Autodesk Inventor part; units mm, degrees
ref_plane "YZ Plane" through (0, 0, 0) normal (1, 0, 0) x (0, 1, 0)
ref_plane "XZ Plane" through (0, 0, 0) normal (0, 1, 0) x (-1, 0, 0)
ref_plane "XY Plane" through (0, 0, 0) normal (0, 0, 1) x (1, 0, 0)
sketch "Sketch1" plane through (0, 0, 0) normal (0, 1, 0) x (-1, 0, 0)
  circle A0 centre (-9, 0) radius 8.5
  circle A1 centre (15, 0) radius 4
  line L0 (10.6066, -10.6066) -> (17.9306, -2.7224)
  line L1 (10.6066, 10.6066) -> (17.9306, 2.7224)
  line L2 (16.6, -2.7713) -> (13.4, -2.7713)
  line L3 (13.4, -2.7713) -> (11.8, 0)
  line L4 (11.8, 0) -> (13.4, 2.7713)
  line L5 (13.4, 2.7713) -> (16.6, 2.7713)
  line L6 (16.6, 2.7713) -> (18.2, 0)
  line L7 (18.2, 0) -> (16.6, -2.7713)
  line L8 (15, -2.7713) -> (15, 2.7713)
  line L9 (11.8, 0) -> (15, 0)
  circle A2 centre (-9, 0) radius 6
  circle A3 centre (-9, -6) radius 1.2
  circle A4 centre (-15, 0) radius 1.2
  circle A5 centre (-9, 6) radius 1.2
  circle A6 centre (-3, 0) radius 1.2
  circle A7 centre (15, 0) radius 1.65
  line L10 (11, 0) -> (-29, 0)
  circle A8 centre (-33, 0) radius 4
  line L11 (-28.6066, -10.6066) -> (-35.9306, -2.7224)
  line L12 (-28.6066, 10.6066) -> (-35.9306, 2.7224)
  line L13 (-31.4, -2.7713) -> (-34.6, -2.7713)
  line L14 (-34.6, -2.7713) -> (-36.2, 0)
  line L15 (-36.2, 0) -> (-34.6, 2.7713)
  line L16 (-36.2, 0) -> (-33, 0)
  line L17 (-33, -2.7713) -> (-33, 2.7713)
  line L18 (-34.6, 2.7713) -> (-31.4, 2.7713)
  line L19 (-29.8, 0) -> (-31.4, -2.7713)
  line L20 (-31.4, 2.7713) -> (-29.8, 0)
  circle A9 centre (-33, 0) radius 1.65
  line L21 (-28.6066, -10.6066) -> (10.6066, -10.6066)
  line L22 (-28.6066, 10.6066) -> (10.6066, 10.6066)
  dimension "d49" = 4
  dimension "d55" = 8
  dimension "d22" = 3.2
  dimension "d34" = 12
  dimension "d35" = 2.4
  dimension "d36" = 2.4
  dimension "d37" = 2.4
  dimension "d38" = 2.4
  dimension "d43" = 3.3
  dimension "d54" = 40
  dimension "d56" = 3.2
  dimension "d57" = 3.2
  dimension "d58" = 120
  dimension "d59" = 3.2
  dimension "d60" = 120
  dimension "d61" = 3.3
extrude "Extrusion1" add sketch "Sketch1" along normal blind 10 contours L10 A6 A2 A5 A4 A0 | L10 A1 L0 L21 L11 A8 A0 | A0 L10 A8 L12 L22 L1 A1 | A0 L10 A4 A2 A3 A6 | A1 | L10 A2 A6 | A6 A2 L10 | L10 A2 A4 | A4 A2 L10 | A8 | A6 L10 A4 A2 A5 | A2 L10 A6 | A6 L10 A2 | A2 A3 A4 L10 A6 | A4 L10 A2 | A2 L10 A4 | A5 A2 | A2 A5 | A3 A2 | A2 A3 | L2 L8 A7 L5 L6 L7 | L2 L3 L9 A7 L8 | A7 L9 L8 | L8 A7 | L4 L5 L8 A7 L9 | L9 A7 L8 | L13 L17 A9 L18 L20 L19 | L13 L14 L16 A9 L17 | A9 L16 L17 | L17 A9 | L15 L18 L17 A9 L16 | L16 A9 L17
extrude "Extrusion2" cut sketch "Sketch1" along normal blind 2.5 contours L10 A6 A2 A5 A4 A0 | A0 L10 A4 A2 A3 A6 | L10 A2 A6 | A6 A2 L10 | L10 A2 A4 | A4 A2 L10 | A6 L10 A4 A2 A5 | A2 L10 A6 | A6 L10 A2 | A2 A3 A4 L10 A6 | A4 L10 A2 | A2 L10 A4 | A5 A2 | A2 A5 | A3 A2 | A2 A3 | L2 L8 A7 L5 L6 L7 | L2 L3 L9 A7 L8 | A7 L9 L8 | L8 A7 | L4 L5 L8 A7 L9 | L9 A7 L8 | L13 L17 A9 L18 L20 L19 | L13 L14 L16 A9 L17 | A9 L16 L17 | L17 A9 | L15 L18 L17 A9 L16 | L16 A9 L17
extrude "Extrusion3" cut sketch "Sketch1" along normal blind 10 contours L10 A2 A6 | A6 A2 L10 | L10 A2 A4 | A4 A2 L10 | A2 L10 A6 | A6 L10 A2 | A4 L10 A2 | A2 L10 A4 | A5 A2 | A2 A5 | A3 A2 | A2 A3 | A7 L9 L8 | L8 A7 | L9 A7 L8 | A9 L16 L17 | L17 A9 | L16 A9 L17
fillet "Fillet1" radius 0.3 20 edges at (-19, 0, 0) (-14.2686, 0, 6.6645) (-14.2686, 0, -6.6645) (-19, 10, 0) (-14.2686, 10, 6.6645) (-14.2686, 10, -6.6645) (9, 10, 10.6066) (9, 0, 10.6066) (9, 10, -10.6066) (9, 0, -10.6066) (-10.6066, 5, -10.6066) (-10.6066, 5, 10.6066) (37, 0, 0) (32.2686, 0, -6.6645) (32.2686, 0, 6.6645) (37, 10, 0) (32.2686, 10, -6.6645) (32.2686, 10, 6.6645) (28.6066, 5, -10.6066) (28.6066, 5, 10.6066)
sketch "Sketch2" plane through (0, 10, 0) normal (0, 1, 0) x (1, 0, 0)
  circle A0 centre (3, 0) radius 1.2
  circle A1 centre (3, 0) radius 2
  circle A2 centre (9, 6) radius 1.2
  circle A3 centre (9, 6) radius 2
  circle A4 centre (15, 0) radius 1.2
  circle A5 centre (15, 0) radius 2
  circle A6 centre (9, -6) radius 1.2
  circle A7 centre (9, -6) radius 2
  point P0 (0, 0)
  dimension "d22" = 3.2
  dimension "d43" = 3.3
  dimension "d48" = 4
  dimension "d49" = 4
  dimension "d50" = 4
  dimension "d51" = 4
extrude "Extrusion5" cut sketch "Sketch2" against normal blind 2 contours A0 | A1 | A2 | A3 | A4 | A5 | A6 | A7
properties part number "neck_v2"
Input: part model. Units: mm. Frame: model coordinates. A direction names the side the tool comes from. Coordinates: 2 decimals unless noted, no trailing zeros. Write each loop counter-clockwise with the first axis right and the second up, starting at its lowest first coordinate (ties: lowest second). Pieces come first, ordered by that corner, then holes.
1) Section D-D on y = 8.5. Output: boundary loops of the cut face in (x, z).
2) Section B-B on y = 6.25. Output: boundary loops of the cut face in (x, z), and give its area (4 significant figures).
3) Section A-A on x = 9. Output: boundary loops of the cut face in (y, z), and give its area (3 significant figures).
4) Material intervals for line 1 along Z through (x, y) = (9, 5.5); line 2 along Z through (x, y) = (3, 6.2); line 3 along Y through (x, z) = (4, -5.75), sorted ascending.
5) Mould query, pull axis X, two halves, no side actions, for faces 1 (the cylindrical face through (7.4, 9, 7.2)), 2 (the cylindrical face through (-14.298, 9.914, -6.501)), 3 (the cylindrical face through (32.298, 9.914, 6.501)). Classes: pulls with the +X half, pulls with the -X half, needs draft (parallel to the pull), parting line crosses it, or undercut.
6) Set-up query: faces 4 (the cylindrical face through (-14.2, 9.91, 6.61)), 5 (the flat face through (-15, 1, -2.771)), 6 (the cylindrical face through (3, 9, 2)). Return all of +Z, -Z, +X, -X, +Y, -Y with unobstructed straight access to the full face (end or side cutting, diameter ignored); none if empty.
7) Pin query (flat end, axial travel): pin 1 Ø2 at (x, y) = (33, 1) entering from +Z; pin 2 Ø3.5 at (x, z) = (3, 0) entering from +Y; pin 3 Ø5 at (y, z) = (5, -2.5) entering from +X; pin 4 Ø4 at (x, z) = (-15, 0) entering from -Y. Return the tip coordinate at first contact, or that it passes through.
8) Section C-C on x = 15. Output: boundary loops of the cut face in (y, z), and give its area (3 significant figures).
Check result:
1. outline: (-17.93, -2.72) - (-10.7, -10.51) arc R0.3 ccw to (-10.48, -10.61) - (28.48, -10.61) arc R0.3 ccw to (28.7, -10.51) - (35.93, -2.72) arc R4 ccw to (35.93, 2.72) - (28.7, 10.51) arc R0.3 ccw to (28.48, 10.61) - (-10.48, 10.61) arc R0.3 ccw to (-10.7, 10.51) - (-17.93, 2.72) arc R4 ccw to start; hole circle Ø3.3 at (-15, 0); hole circle Ø4 at (3, 0); hole circle Ø4 at (9, -6); hole circle Ø4 at (9, 6); hole circle Ø4 at (15, 0); hole circle Ø3.3 at (33, 0)
2. outline: (-17.93, -2.72) - (-10.7, -10.51) arc R0.3 ccw to (-10.48, -10.61) - (28.48, -10.61) arc R0.3 ccw to (28.7, -10.51) - (35.93, -2.72) arc R4 ccw to (35.93, 2.72) - (28.7, 10.51) arc R0.3 ccw to (28.48, 10.61) - (-10.48, 10.61) arc R0.3 ccw to (-10.7, 10.51) - (-17.93, 2.72) arc R4 ccw to start; hole circle Ø3.3 at (-15, 0); hole circle Ø2.4 at (3, 0); hole circle Ø2.4 at (9, -6); hole circle Ø2.4 at (9, 6); hole circle Ø2.4 at (15, 0); hole circle Ø3.3 at (33, 0)
2. area: 1,000 mm2
3. outline: (0, -10.31) arc R0.3 ccw to (0.3, -10.61) - (9.7, -10.61) arc R0.3 ccw to (10, -10.31) - (10, -8) - (8, -8) - (8, -7.2) - (2.5, -7.2) - (2.5, -8.5) - (0, -8.5) - close; (0, 8.5) - (2.5, 8.5) - (2.5, 7.2) - (8, 7.2) - (8, 8) - (10, 8) - (10, 10.31) arc R0.3 ccw to (9.7, 10.61) - (0.3, 10.61) arc R0.3 ccw to (0, 10.31) - close; (2.5, -4.8) - (8, -4.8) - (8, -4) - (10, -4) - (10, 4) - (8, 4) - (8, 4.8) - (2.5, 4.8) - close
3. area: 127 mm2
4. line 1: z = -10.61 to -7.2, -4.8 to 4.8, 7.2 to 10.61
4. line 2: z = -10.61 to -1.2, 1.2 to 10.61
4. line 3: y = 2.5 to 10
5. face 1: undercut
5. face 2: pulls with the -X half
5. face 3: pulls with the +X half
6. face 4: +Z, -X, +Y
6. face 5: -Y
6. face 6: +Y
7. pin 1: stops at z = 6.95
7. pin 2: stops at y = 8
7. pin 3: stops at x = 37
7. pin 4: stops at y = 2.5
8. outline: (0, -10.31) arc R0.3 ccw to (0.3, -10.61) - (9.7, -10.61) arc R0.3 ccw to (10, -10.31) - (10, -2) - (8, -2) - (8, -1.2) - (2.5, -1.2) - (2.5, -6.02) - (0, -6.02) - close; (0, 6.02) - (2.5, 6.02) - (2.5, 1.2) - (8, 1.2) - (8, 2) - (10, 2) - (10, 10.31) arc R0.3 ccw to (9.7, 10.61) - (0.3, 10.61) arc R0.3 ccw to (0, 10.31) - close
8. area: 161 mm2
